Build history of the part. All positions in model axes, mm. Face numbers are marked on the shaded views. A direction names the side the tool comes from. Round coordinates to 2 decimals unless told otherwise and drop trailing zeros. Write each loop counter-clockwise with the first axis right and the second up, starting at its lowest first coordinate (ties: lowest second). Pieces come first, ordered by that corner, then holes. Notation, with made-up numbers: M -13.75,58.25 L 35.25,58.25 A19 ccw 35.25,95.25 Z; hole C 2.25,75 d7. An arc over 180 degrees is marked long. Write item = value, one per line. Start each with the question number.
Q1. Band-saw the part on A-A on z = -61.5. Write the cut outline in (x, y), plus the area to 3 significant figures.
Q2. Drop flat-ended pins along their axis: P1, Ø1.8, axis at y = 31, z = -62.5, coming from the +X side; P2, Ø18.5, axis at y = -3.5, z = -65.5, coming from the +X side; P3, Ø2, axis at x = -4, z = -23.5, coming from the +Y side. Give the stop position or say it passes through.
Q3. Tool access for the marked faces 1, 2, 3 and 4: list every direction of +Z, -Z, +X, -X, +Y, -Y with a clear straight run to the whole face (end or side of a thin tool).
Q4. Band-saw the part on B-B on x = -10. State how many separate pieces and enclosed holes the cut face has, plus the area to 3 significant figures.
Q5. Probe L1, parallel to X at y = 2, z = -39.5; L2, parallel to Z at x = -13.25, y = -19; L3, parallel to Y at x = -13, z = -60. List the from-to ranges inside material, lowest first.
```python
from build123d import *

# Parameters (mm, degrees)
F5_DEPTH  = 3
F6_W      = 2.25
F6_H      = 23
F7_DEPTH  = 20
F13_DEPTH = 35


with BuildPart() as f3:
    # F2 (on offset) → F3 section 0
    with BuildSketch(Plane.XY.offset(-50)):
        with BuildLine():
            Line((-3.5000038791, 20.4748884357), (-3.5000038791, 27.4999761514))
            ThreePointArc((-3.5000038791, 27.4999761514), (-2.9142174415, 28.9141897138), (-1.5000038791, 29.4999761514))
            Line((-1.5000038791, 29.4999761514), (-3.8791e-06, 29.4999761514))
            Line((-3.8791e-06, 29.4999761514), (-3.8791e-06, 31.7499761514))
            Line((-3.8791e-06, 31.7499761514), (-1.5000038791, 31.7499761514))
            ThreePointArc((-1.5000038791, 31.7499761514), (-4.5052076991, 30.5051799715), (-5.7500038791, 27.4999761514))
            Line((-5.7500038791, 27.4999761514), (-5.7500038791, 20.6592524712))
            Line((-5.7500038791, 20.6592524712), (-12.4557502015, 18.5853103096))
            ThreePointArc((-12.4557502015, 18.5853103096), (-14.6204878997, 17.0475208172), (-15.4500038791, 14.5250638671))
            Line((-15.4500038791, 14.5250638671), (-15.4500038791, 0.6637059035))
            ThreePointArc((-15.4500038791, 0.6637059035), (-15.4670184988, 0.1504446566), (-15.5179876488, -0.3605629272))
            Line((-15.5179876488, -0.3605629272), (-16.1221071747, -4.8914593715))
            ThreePointArc((-16.1221071747, -4.8914593715), (-16.2137025969, -5.8872580453), (-16.223770689, -6.887209721))
            Line((-16.223770689, -6.887209721), (-16.223770689, -22.3192218691))
            Line((-16.223770689, -22.3192218691), (-13.9748350221, -22.3192218691))
            Line((-13.9748350221, -22.3192218691), (-13.9748350221, -6.8180117005))
            ThreePointArc((-13.9748350221, -6.8180117005), (-13.9666161714, -6.0017246183), (-13.8918443982, -5.1888277417))
            Line((-13.8918443982, -5.1888277417), (-13.2877248723, -0.6579312974))
            ThreePointArc((-13.2877248723, -0.6579312974), (-13.2219582271, 0.0014333268), (-13.2000038791, 0.6637059035))
            Line((-13.2000038791, 0.6637059035), (-13.2000038791, 14.5250638671))
            ThreePointArc((-13.2000038791, 14.5250638671), (-12.8096434182, 15.7121024319), (-11.790943325, 16.4357680754))
            Line((-11.790943325, 16.4357680754), (-4.9090644333, 18.5641842274))
            ThreePointArc((-4.9090644333, 18.5641842274), (-3.89036434, 19.2878498709), (-3.5000038791, 20.4748884357))
        make_face()
    # F0 (on Top) → F3 section 1
    with BuildSketch(Plane.XY):
        with BuildLine():
            Line((-3.5, 20.4749122843), (-3.5, 27.5))
            ThreePointArc((-3.5, 27.5), (-2.9142135624, 28.9142135624), (-1.5, 29.5))
            Line((-1.5, 29.5), (0, 29.5))
            Line((0, 29.5), (0, 31.75))
            Line((0, 31.75), (-1.5, 31.75))
            ThreePointArc((-1.5, 31.75), (-4.50520382, 30.50520382), (-5.75, 27.5))
            Line((-5.75, 27.5), (-5.75, 20.6592763198))
            Line((-5.75, 20.6592763198), (-12.4557463224, 18.5853341582))
            ThreePointArc((-12.4557463224, 18.5853341582), (-14.6204840206, 17.0475446658), (-15.45, 14.5250877157))
            Line((-15.45, 14.5250877157), (-15.45, 0.6637297521))
            ThreePointArc((-15.45, 0.6637297521), (-15.4670146197, 0.1504685052), (-15.5179837697, -0.3605390786))
            Line((-15.5179837697, -0.3605390786), (-16.1221032956, -4.8914355229))
            ThreePointArc((-16.1221032956, -4.8914355229), (-16.2136987178, -5.8872341967), (-16.2237668099, -6.8871858724))
            Line((-16.2237668099, -6.8871858724), (-15.7489356669, -22.3191980205))
            Line((-15.7489356669, -22.3191980205), (-13.5, -22.25))
            Line((-13.5, -22.25), (-13.974831143, -6.8179878519))
            ThreePointArc((-13.974831143, -6.8179878519), (-13.9666122923, -6.0017007697), (-13.8918405191, -5.1888038931))
            Line((-13.8918405191, -5.1888038931), (-13.2877209932, -0.6579074488))
            ThreePointArc((-13.2877209932, -0.6579074488), (-13.221954348, 0.0014571754), (-13.2, 0.6637297521))
            Line((-13.2, 0.6637297521), (-13.2, 14.5250877157))
            ThreePointArc((-13.2, 14.5250877157), (-12.8096395391, 15.7121262805), (-11.7909394458, 16.435791924))
            Line((-11.7909394458, 16.435791924), (-4.9090605542, 18.564208076))
            ThreePointArc((-4.9090605542, 18.564208076), (-3.8903604609, 19.2878737195), (-3.5, 20.4749122843))
        make_face()
    loft()

    # F4 (on face) → F5 (join)
    with BuildSketch(Plane(origin=(0, 0, -50), x_dir=(1, 0, 0), z_dir=(0, 0, -1))):
        with BuildLine():
            Line((-13.2000038791, -0.6637059035), (-15.4500038791, -0.6637059035))
            Line((-15.4500038791, -0.6637059035), (-15.4500038791, -14.5250638671))
            ThreePointArc((-15.4500038791, -14.5250638671), (-14.6204878997, -17.0475208172), (-12.4557502015, -18.5853103096))
            Line((-12.4557502015, -18.5853103096), (-5.7500038791, -20.6592524712))
            Line((-5.7500038791, -20.6592524712), (-5.7500038791, -27.4999761514))
            ThreePointArc((-5.7500038791, -27.4999761514), (-4.5052076991, -30.5051799715), (-1.5000038791, -31.7499761514))
            Line((-1.5000038791, -31.7499761514), (-3.8791e-06, -31.7499761514))
            Line((-3.8791e-06, -31.7499761514), (-3.8791e-06, -29.4999761514))
            Line((-3.8791e-06, -29.4999761514), (-1.5000038791, -29.4999761514))
            ThreePointArc((-1.5000038791, -29.4999761514), (-2.9142174415, -28.9141897138), (-3.5000038791, -27.4999761514))
            Line((-3.5000038791, -27.4999761514), (-3.5000038791, -20.4748884357))
            ThreePointArc((-3.5000038791, -20.4748884357), (-3.89036434, -19.2878498709), (-4.9090644333, -18.5641842274))
            Line((-4.9090644333, -18.5641842274), (-11.790943325, -16.4357680754))
            ThreePointArc((-11.790943325, -16.4357680754), (-12.8096434182, -15.7121024319), (-13.2000038791, -14.5250638671))
            Line((-13.2000038791, -14.5250638671), (-13.2000038791, -0.6637059035))
        make_face()
    extrude(amount=F5_DEPTH)

    # F6 (on face) → F7 (join)
    with BuildSketch(Plane(origin=(0, 0, -53), x_dir=(1, 0, 0), z_dir=(0, 0, -1))):
        with BuildLine():
            Line((-13.2000038791, -14.5250638671), (-13.2000038791, -0.6637059035))
            Line((-13.2000038791, -0.6637059035), (-15.4500038791, -0.6637059035))
            Line((-15.4500038791, -0.6637059035), (-15.4500038791, -14.5250638671))
            ThreePointArc((-15.4500038791, -14.5250638671), (-14.6204878997, -17.0475208172), (-12.4557502015, -18.5853103096))
            Line((-12.4557502015, -18.5853103096), (-5.7500038791, -20.6592524712))
            Line((-5.7500038791, -20.6592524712), (-5.7500038791, -27.4999761514))
            ThreePointArc((-5.7500038791, -27.4999761514), (-4.5052076991, -30.5051799715), (-1.5000038791, -31.7499761514))
            Line((-1.5000038791, -31.7499761514), (-3.8791e-06, -31.7499761514))
            Line((-3.8791e-06, -31.7499761514), (-3.8791e-06, -29.4999761514))
            Line((-3.8791e-06, -29.4999761514), (-1.5000038791, -29.4999761514))
            ThreePointArc((-1.5000038791, -29.4999761514), (-2.9142174415, -28.9141897138), (-3.5000038791, -27.4999761514))
            Line((-3.5000038791, -27.4999761514), (-3.5000038791, -20.4748884357))
            ThreePointArc((-3.5000038791, -20.4748884357), (-3.89036434, -19.2878498709), (-4.9090644333, -18.5641842274))
            Line((-4.9090644333, -18.5641842274), (-11.790943325, -16.4357680754))
            ThreePointArc((-11.790943325, -16.4357680754), (-12.8096434182, -15.7121024319), (-13.2000038791, -14.5250638671))
        make_face()
        with Locations((-14.3250038791, 10.8362940965)):
            Rectangle(F6_W, F6_H)
    extrude(amount=F7_DEPTH)

    # F10: sweep along a path in F10_path
    with BuildLine(Plane(origin=(-15.4500038791, -22.3362940965, -73), x_dir=(0, 0, -1), z_dir=(0, 1, 0))) as f10_path:
        Line((0, 0), (-20, 0))
    # F8 (on face) → F10 (sweep)
    with BuildSketch(Plane(origin=(0, 0, -73), x_dir=(1, 0, 0), z_dir=(0, 0, -1))):
        Polygon((-15.4500038791, 22.3362940965), (-13.2000038791, 22.3362940965), (0, 23.2500238486), (0, 25.5000238486), (-15.4500038791, 24.4305447527), align=None)
    sweep(path=f10_path.line)

    # F11: sweep along a path in F11_path
    with BuildLine(Plane(origin=(-13.9748350221, -22.3192218691, -50), x_dir=(-0.0094962722, 0, -0.9999549094), z_dir=(-0.9999549094, 0, 0.0094962722))) as f11_path:
        add(Plane(origin=(-13.9748350221, -22.3192218691, -50), x_dir=(-0.0094962722, 0, -0.9999549094), z_dir=(-0.9999549094, 0, 0.0094962722)) * Edge.make_bspline(
            [(0, 0), (-50.0022546321, -0.0692218691)],
            knots=[0, 0, 1, 1], degree=1))
    # F9 (on face) → F11 (sweep)
    with BuildSketch(Plane(origin=(0, 0, -50), x_dir=(1, 0, 0), z_dir=(0, 0, -1))):
        Polygon((-16.223770689, 22.3192218691), (-13.9748350221, 22.3192218691), (0, 23.2500238486), (0, 25.649815511), (-16.223770689, 24.5692218691), align=None)
    sweep(path=f11_path.line)

    # F12 (on face) → F13 (cut)
    with BuildSketch(Plane.XY):
        with BuildLine():
            add(Edge.make_bspline(
                [(-13.5, -22.25), (0.4748350221, -23.1808019795)],
                knots=[0, 0, 14.0057990211, 14.0057990211], degree=1))
            Line((-13.5, -22.25), (-15.7489356669, -22.3191980205))
            add(Edge.make_bspline(
                [(-15.7489356669, -24.5), (-15.7489356669, -22.3191980205)],
                knots=[0, 0, 2.1808019795, 2.1808019795], degree=1))
            add(Edge.make_bspline(
                [(0.4748350221, -25.5805936419), (-15.7489356669, -24.5)],
                knots=[0, 0, 16.2597176479, 16.2597176479], degree=1))
            add(Edge.make_bspline(
                [(0.4748350221, -23.1808019795), (0.4748350221, -25.5805936419)],
                knots=[0, 0, 2.3997916625, 2.3997916625], degree=1))
        make_face()
        with BuildLine():
            Line((1.4795829775, -22.3191980205), (-13.5, -22.25))
            add(Edge.make_bspline(
                [(-13.5, -22.25), (0.4748350221, -23.1808019795)],
                knots=[0, 0, 14.0057990211, 14.0057990211], degree=1))
            add(Edge.make_bspline(
                [(0.4748350221, -23.1808019795), (0.4748350221, -25.5805936419)],
                knots=[0, 0, 2.3997916625, 2.3997916625], degree=1))
            add(Edge.make_bspline(
                [(0.4748350221, -25.5805936419), (-15.7489356669, -24.5)],
                knots=[0, 0, 16.2597176479, 16.2597176479], degree=1))
            add(Edge.make_bspline(
                [(-15.7489356669, -24.5), (-15.7489356669, -22.3191980205)],
                knots=[0, 0, 2.1808019795, 2.1808019795], degree=1))
            Line((-15.7489356669, -22.3191980205), (-16.8508291245, -22.3191980205))
            Line((-16.8508291245, -22.3191980205), (-16.8508291245, -25.5727563053))
            Line((-16.8508291245, -25.5727563053), (1.4795829775, -27.0518492907))
            Line((1.4795829775, -27.0518492907), (1.4795829775, -22.3191980205))
        make_face()
    extrude(amount=-F13_DEPTH, mode=Mode.SUBTRACT)


solid = f3.part
```
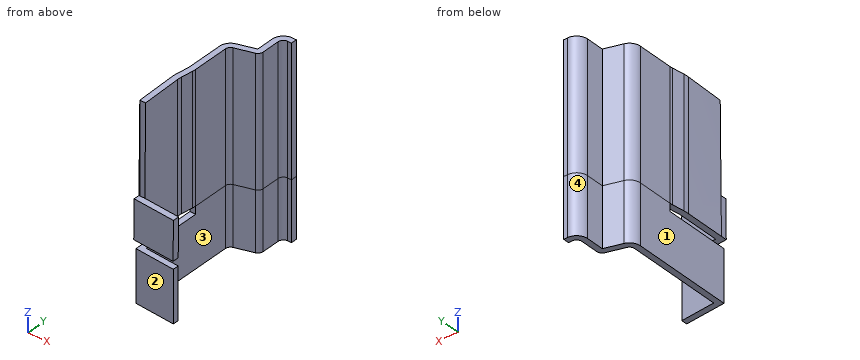
Conclusion:
q1.outline = M -15.45,-24.43 L 0,-25.5 L 0,-23.25 L -13.2,-22.34 L -13.2,14.53 A2 cw -11.79,16.44 L -4.91,18.56 A2 ccw -3.5,20.47 L -3.5,27.5 A2 cw -1.5,29.5 L 0,29.5 L 0,31.75 L -1.5,31.75 A4.25 ccw -5.75,27.5 L -5.75,20.66 L -12.46,18.59 A4.25 ccw -15.45,14.53 Z
q1.area = 175 mm^2
q2.P1 = 0
q2.P2 = -13.2
q2.P3 = 31.48
q3.face_1 = -Z, -X, +Y, -Y
q3.face_2 = -Z, -X, -Y
q3.face_3 = +Z, -Z, +X
q3.face_4 = +Z, -Z, -X, +Y
q4.separate_pieces = 3
q4.enclosed_holes = 0
q4.area = 253 mm^2
q5.L1 = -15.45 to -13.2
q5.L2 = -73 to -53
q5.L3 = -24.6 to -22.35, 15.4 to 18.38
